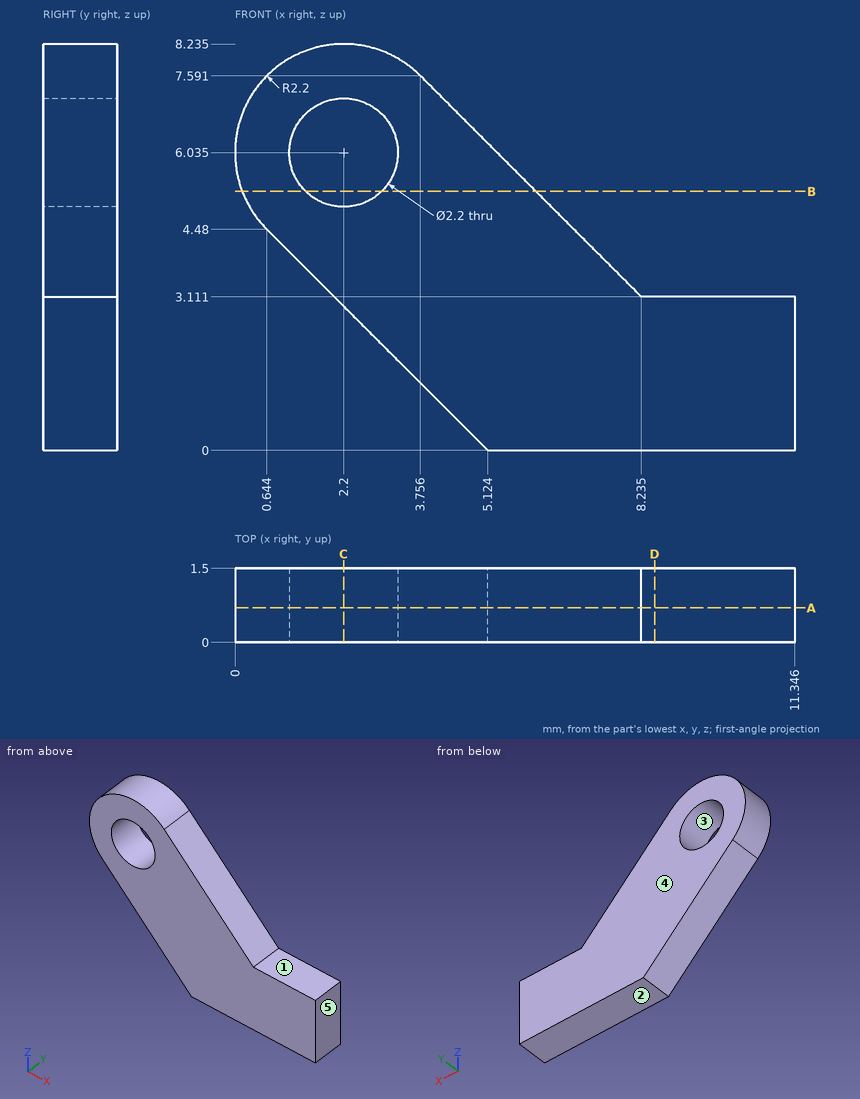
For this review, use the dimensioned drawing (mm, ordinates from the lowest corner) and the shaded views. A direction names the side the tool comes from. Give positions to 0.01 mm unless a question says otherwise; leave off trailing zeros. Order: outer loops, then holes, each group sorted by start corner. A loop starts at its lowest first (then second) coordinate and runs counter-clockwise, first axis right, second up.
1) The part is to be moulded in two halves that separate along X. For the marked faces 3, 4 and 5, say which applies: released by +X, released by -X, zero draft, split by the parting line, or undercut.
2) For the marked faces 1 and 2, list the 3-axis set-ups (+Z, -Z, +X, -X, +Y, -Y) from which the entire face can be reached by the end or side of a thin tool; tool diameter is ignored.
3) Take a section at D-D (x = 8.5). Give the boundary of the cut face in (y, z).
4) Take a section at C-C (x = 2.2). Give the boundary of the cut face in (y, z) (1 decimal).
5) Take a section at B-B (z = 5.25). Give the boundary of the cut face in (x, y) (1 decimal).
6) Take a section at A-A (y = 0.7). Give the boundary of the cut face in (x, z) (1 decimal), then the cut area to 3 significant figures.
7) Wall thickness on line 1 (X direction, y = 0.75, z = 6.75) (1 decimal); line 2 (Z direction, x = 2, y = 1.3) (1 decimal); line 3 (Z direction, x = 2.5, y = 0.3) (1 decimal): over which ranges is each line inside the solid? List them lowest first.
Derived:
1. face 3: undercut
1. face 4: zero draft
1. face 5: released by +X
2. face 1: +Z, +X, +Y, -Y
2. face 2: -Z, +X, -X, +Y, -Y
3. outline: (0, 0) - (1.5, 0) - (1.5, 3.11) - (0, 3.11) - close
4. outline: (0, 2.9) - (1.5, 2.9) - (1.5, 4.9) - (0, 4.9) - close; (0, 7.1) - (1.5, 7.1) - (1.5, 8.2) - (0, 8.2) - close
5. outline: (0.1, 0) - (1.4, 0) - (1.4, 1.5) - (0.1, 1.5) - close; (3, 0) - (6.1, 0) - (6.1, 1.5) - (3, 1.5) - close
6. outline: (0.6, 4.5) - (5.1, 0) - (11.3, 0) - (11.3, 3.1) - (8.2, 3.1) - (3.8, 7.6) arc R2.2 ccw to start; hole circle Ø2.2 at (2.2, 6)
6. area: 46.2 mm2
7. line 1: x = 0.1 to 1.4, 3 to 4.6
7. line 2: z = 3.1 to 5, 7.1 to 8.2
7. line 3: z = 2.6 to 5, 7.1 to 8.2
